Part model, mm, in its own coordinate system. Face numbers are marked on the shaded views. A direction names the side the tool comes from. Give positions to 0.01 mm unless a question says otherwise; leave off trailing zeros. Write each loop counter-clockwise with the first axis right and the second up, starting at its lowest first coordinate (ties: lowest second). Pieces come first, ordered by that corner, then holes. Notation, with made-up numbers: M -24,23 L 21,23 A23 cw 21,59 Z; hole C -13.75,71.5 d8. An arc over 180 degrees is marked long. Use a Markdown table: item, result.
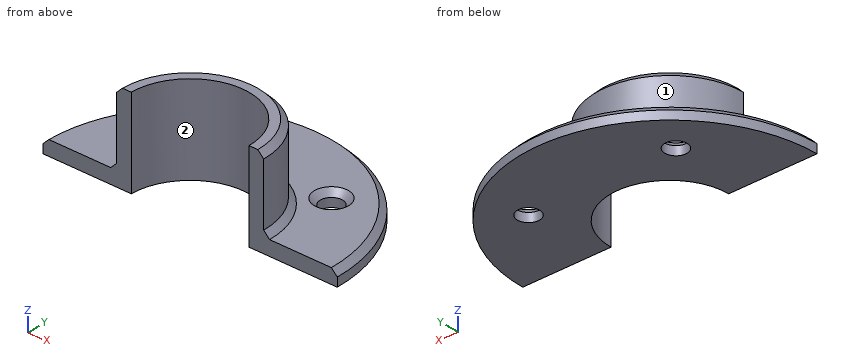
```python
from build123d import *

# Parameters (mm, degrees)
F0_R     = 2.38125
F1_DEPTH = 3.175
F2_DEPTH = 19.05
F3_SIZE  = 1.27


with BuildPart() as f1:
    # F0 (on Top) → F1 (new body)
    with BuildSketch(Plane.XY):
        with BuildLine():
            Line((15.875, 0), (31.75, 0))
            ThreePointArc((31.75, 0), (0, 31.75), (-31.75, 0))
            Line((-31.75, 0), (-15.875, 0))
            ThreePointArc((-15.875, 0), (0, 15.875), (15.875, 0))
        make_face()
        with Locations((-15.9058814723, 16.4189687431)):
            Circle(F0_R, mode=Mode.SUBTRACT)
        with Locations((15.9058814723, 16.4189687431)):
            Circle(F0_R, mode=Mode.SUBTRACT)
    extrude(amount=F1_DEPTH)

    # F0 (on Top) → F2 (join)
    with BuildSketch(Plane.XY):
        with BuildLine():
            Line((12.7, 0), (15.875, 0))
            ThreePointArc((15.875, 0), (0, 15.875), (-15.875, 0))
            Line((-15.875, 0), (-12.7, 0))
            ThreePointArc((-12.7, 0), (0, 12.7), (12.7, 0))
        make_face()
    extrude(amount=F2_DEPTH)

    # F3
    f3_edges = [f1.edges().sort_by_distance(p)[0] for p in [
        (-18.287131, 16.418969, 3.175),
        (13.524631, 16.418969, 3.175),
        (0, 31.75, 3.175),
        (0, 15.875, 19.05),
        (0, 15.875, 3.175),
    ]]
    chamfer(f3_edges, length=F3_SIZE)


solid = f1.part
```
1. Drop flat-ended pins along their axis: P1, Ø4, axis at x = -6, y = 24, coming from the +Z side (3 decimals); P2, Ø8, axis at x = -14.5, z = 10.5, coming from the +Y side; P3, Ø5, axis at x = -5.5, y = 7.5, coming from the -Z side; P4, Ø6, axis at y = 5.5, z = 7, coming from the +X side. Give the stop position or say it passes through.
Findings below:
| item | result |
|---|---|
| P1 | z = 3.175 |
| P2 | y = 11.91 |
| P3 | through |
| P4 | x = 15.68 |
2. Cut at B-B, the plane z = 9.25. Give the cut face in (x, y) (3 decimals).
Findings below:
| item | result |
|---|---|
| outline | M -15.875,0 L -12.7,0 A12.7 cw 12.7,0 L 15.875,0 A15.875 ccw Z |
3. Tool access for the marked faces 1 and 2: list every direction of +Z, -Z, +X, -X, +Y, -Y with a clear straight run to the whole face (end or side of a thin tool).
Findings below:
| item | result |
|---|---|
| face 1 | +Z, +Y |
| face 2 | +Z, -Z, -Y |
4. Drill centre lines: L1, parallel to Z at x = -9, y = 21.5 (3 decimals); L2, parallel to X at y = 5, z = 13.75; L3, parallel to X at y = 2, z = 11.5. Where is each one in solid material? Low to high.
Findings below:
| item | result |
|---|---|
| L1 | 0 to 3.175 |
| L2 | -15.07 to -11.67, 11.67 to 15.07 |
| L3 | -15.75 to -12.54, 12.54 to 15.75 |
5. Cut at A-A, the plane x = 0. Give the cut face in (y, z) (3 decimals).
Findings below:
| item | result |
|---|---|
| outline | M 12.7,0 L 31.75,0 L 31.75,1.905 L 30.48,3.175 L 17.145,3.175 L 15.875,4.445 L 15.875,17.78 L 14.605,19.05 L 12.7,19.05 Z |
